Could you check a few things on this model? Use its own coordinates, in mm. A direction names the side the tool comes from. Coordinates: 2 decimals unless noted, no trailing zeros. Order: outer loops, then holes, each group sorted by start corner. A loop starts at its lowest first (then second) coordinate and runs counter-clockwise, first axis right, second up.
Autodesk Inventor part; units mm, degrees
ref_plane "YZ Plane" through (0, 0, 0) normal (1, 0, 0) x (0, 1, 0)
ref_plane "XZ Plane" through (0, 0, 0) normal (0, 1, 0) x (-1, 0, 0)
ref_plane "XY Plane" through (0, 0, 0) normal (0, 0, 1) x (1, 0, 0)
sketch "Skizze1" plane through (0, 0, 0) normal (0, 1, 0) x (-1, 0, 0)
  line L0 (-198.8627, 53.5938) -> (99.1639, 53.5938) construction
  line L1 (99.1639, 53.5938) -> (99.1639, -114.0462) construction
  line L2 (99.1639, -114.0462) -> (-198.8627, -114.0462) construction
  line L3 (-198.8627, -114.0462) -> (-198.8627, 53.5938) construction
  circle A0 centre (0.0046, 0.0192) radius 18.7265
  line L4 (-9.419, 18.8182) -> (-23.9308, 8.0268)
  line L5 (-23.9308, 8.0268) -> (-23.9308, -2.2349)
  line L6 (-23.9308, -2.2349) -> (-16.3101, -12.64)
  line L7 (-16.3101, -12.64) -> (-10.5238, -15.9026)
  line L8 (-10.5238, -15.9026) -> (-6.65, -19.5009)
  line L9 (-6.65, -19.5009) -> (-5.075, -19.5009)
  line L10 (-5.075, -19.5009) -> (-4.0313, -20.4704)
  line L11 (-4.0313, -20.4704) -> (8.2132, -20.4099)
  line L12 (8.2132, -20.4099) -> (16.9625, -13.9037)
  line L13 (16.9625, -13.9037) -> (18.4985, -11.1795)
  line L14 (18.4985, -11.1795) -> (22.5122, -8.2399)
  line L15 (22.5122, -8.2399) -> (21.5218, -3.0373)
  line L16 (21.5218, -3.0373) -> (23.1766, 5.5058)
  line L17 (23.1766, 5.5058) -> (19.9087, 11.8258)
  line L18 (19.9087, 11.8258) -> (16.0647, 13.9933)
  line L19 (16.0647, 13.9933) -> (14.1168, 21.4913)
  line L20 (14.1168, 21.4913) -> (7.2513, 30.8655)
  line L21 (7.2513, 30.8655) -> (-10.5238, 24.3271)
  line L22 (-10.5238, 24.3271) -> (-10.5238, 20.9548)
  line L23 (-10.5238, 20.9548) -> (-9.419, 18.8182)
  line L24 (-17.1251, -13.5581) -> (-25.1308, -2.6273)
  line L25 (-25.1308, -2.6273) -> (-25.1308, 8.6299)
  line L26 (-25.1308, 8.6299) -> (-10.9532, 19.1727)
  line L27 (-10.9532, 19.1727) -> (-11.7238, 20.6629)
  line L28 (-11.7238, 20.6629) -> (-12.4385, 27.9461)
  line L29 (-12.4385, 27.9461) -> (8.4751, 34.2404)
  line L30 (8.4751, 34.2404) -> (15.2206, 22.0152)
  line L31 (15.2206, 22.0152) -> (17.098, 14.7883)
  line L32 (17.098, 14.7883) -> (20.8101, 12.6952)
  line L33 (20.8101, 12.6952) -> (24.434, 5.6868)
  line L34 (24.434, 5.6868) -> (22.7438, -3.0393)
  line L35 (22.7438, -3.0393) -> (23.8328, -8.7601)
  line L36 (23.8328, -8.7601) -> (19.4166, -11.9945)
  line L37 (19.4166, -11.9945) -> (17.8827, -14.7148)
  line L38 (17.8827, -14.7148) -> (8.6131, -21.608)
  line L39 (8.6131, -21.608) -> (-4.5001, -21.6727)
  line L40 (-4.5001, -21.6727) -> (-5.5463, -20.7009)
  line L41 (-5.5463, -20.7009) -> (-7.1214, -20.7009)
  line L42 (-7.1214, -20.7009) -> (-11.2367, -16.8783)
  line L43 (-11.2367, -16.8783) -> (-17.1251, -13.5581)
  dimension "d4" = 37.453
  dimension "d29" = 42
  dimension "d45" = 1.2
extrude "Extrusion1" add sketch "Skizze1" along normal blind 10 contours L23 L22 L21 L20 L19 L18 L17 L16 L15 L14 L13 L12 L11 L10 L9 L8 L7 L6 L5 L4 | L24 L25 L26 L27 L28 L29 L30 L31 L32 L33 L34 L35 L36 L37 L38 L39 L40 L41 L42 L43
sketch "Skizze2" plane through (0, 10, 0) normal (0, 1, 0) x (1, 0, 0)
  circle A0 centre (-0.0046, -0.0192) radius 18.7265
  line L0 (-9.9482, -31.8575) -> (-12.8321, -24.0172)
  line L1 (-12.8321, -24.0172) -> (9.0572, -15.9655)
  line L2 (9.0572, -15.9655) -> (11.9411, -23.8058)
  line L3 (11.9411, -23.8058) -> (-9.9482, -31.8575)
  line L4 (-7.2513, -30.8655) -> (10.5238, -24.3271)
  circle A1 centre (-0.0046, -0.0192) radius 18.7265
  circle A2 centre (-0.0046, -0.0192) radius 21
  point P0 (0, 0)
  point P1 (9.9588, -18.4167)
  point P2 (9.1919, -16.3319)
  point P3 (1.714, -18.6666)
  point P4 (-12.3868, -23.8534)
  dimension "d38" = 42
extrude "Extrusion2" add sketch "Skizze2" along normal blind 2.5
sketch "Skizze3" plane through (0, 12.5, 0) normal (0, 1, 0) x (1, 0, 0)
  circle A0 centre (-0.0046, -0.0192) radius 18.7265
  circle A1 centre (-0.0046, -0.0192) radius 21
  point P0 (0, 0)
  dimension "d41" = 42
extrude "Extrusion3" add sketch "Skizze3" along normal blind 4.5 contours A0 | A1
properties part number "01_Objektiv"
Item 1: Thinking about a two-plate mould opening in X: for faces 6 (the face through (-11.37, 11.23, 27.99)), 7 (the face through (-20, 10, 7)), 8 (the face through (0, 10, 0)), 9 (the face through (-17.866, 4.93, -5.606)), which applies, +X half, -X half, draft (parallel to the pull), parting line (faces both ways), or undercut?
Item 2: Suppose I cut it at C-C (x = -5.5). List the corners of the cut face in (y, z) for me (3 decimals), and give its area (3 significant figures).
Item 3: For pin 1 Ø4 at (x, y) = (0, 3) entering from -Z; pin 2 Ø4 at (x, z) = (-0.5, 15.5) entering from -Y; pin 3 Ø8 at (x, y) = (11.5, 11.5) entering from -Z; pin 4 Ø2 at (x, z) = (-18, 16.5) entering from +Y, each with a flat end and sliding along its axis, tell me the tip position at first contact or that it passes through.
Item 4: Which directions (+Z, -Z, +X, -X, +Y, -Y) give clear straight access to the entire face, cutting with the end or side of a thin tool? Please do faces 1 (the face through (25.131, 5, 3)), 2 (the face through (10.95, 11.23, 21.11)), 3 (the face through (-23.6, 4.93, 1.38)), 4 (the face through (12.076, 4.93, 24.254)), 5 (the face through (-18.66, 4.93, -13.34)).
Item 5: Suppose I cut it at B-B (z = 23). List the corners of the cut face in (x, y) for me, and give its area (3 significant figures).
Item 6: Suppose I cut it at D-D (z = 6.5). List the corners of the cut face in (x, y) for me, and give its area (3 significant figures).
Item 7: Suppose I cut it at A-A (y = 8.5). List the corners of the cut face in (x, z) for me.
Item 8: I need wall thicknesses on line 1 (Y direction, x = -3.5, z = 1); line 2 (Z direction, x = -0.5, y = 4.25); line 3 (Y direction, x = 20.5, z = 9.5). Which ranges of each line are inside material? Lowest first, please.
Geometry results:
1. face 6: -X half
1. face 7: draft
1. face 8: undercut
1. face 9: undercut
2. outline: (0, -21.623) - (10, -21.623) - (10, -20.249) - (17, -20.249) - (17, 20.287) - (10, 20.287) - (10, 21.32) - (12.5, 21.32) - (12.5, 30.221) - (10, 30.221) - (10, 33.345) - (0, 33.345) - (0, 17.921) - (10, 17.921) - (10, -17.883) - (0, -17.883) - close
2. area: 498 mm2
3. pin 1: stops at z = -21.66
3. pin 2: stops at y = 10
3. pin 3: stops at z = -20.08
3. pin 4: passes through
4. face 1: +Z, -Z, +X, +Y, -Y
4. face 2: +X, +Y
4. face 3: -X, +Y, -Y
4. face 4: +X, +Y, -Y
4. face 5: -Z, -X, +Y, -Y
5. outline: (-14.68, 0) - (11.95, 0) - (11.95, 10) - (11.64, 10) - (11.64, 12.5) - (-10.07, 12.5) - (-10.07, 10) - (-14.68, 10) - close
5. area: 321 mm2
6. outline: (-24.01, 0) - (-17.57, 0) - (-17.57, 10) - (17.56, 10) - (17.56, 0) - (25.13, 0) - (25.13, 10) - (19.97, 10) - (19.97, 17) - (-19.98, 17) - (-19.98, 10) - (-24.01, 10) - close
6. area: 420 mm2
7. outline: (-24.43, 5.69) - (-22.74, -3.04) - (-23.83, -8.76) - (-19.42, -11.99) - (-17.88, -14.71) - (-8.61, -21.61) - (4.5, -21.67) - (5.55, -20.7) - (7.12, -20.7) - (11.24, -16.88) - (17.13, -13.56) - (25.13, -2.63) - (25.13, 8.63) - (10.95, 19.17) - (11.72, 20.66) - (12.44, 27.95) - (-8.48, 34.24) - (-15.22, 22.02) - (-17.1, 14.79) - (-20.81, 12.7) - close; hole circle Ø37.45 at (0, 0.02)
8. line 1: y = 10 to 17
8. line 2: z = -21.65 to -18.7, 18.74 to 31.84
8. line 3: y = 0 to 10
